Check sheet for the modelled part. Datum: model origin and axes. Units: mm. Face numbers are marked on the shaded views. A direction names the side the tool comes from. Round coordinates to 2 decimals unless told otherwise and drop trailing zeros. Write each loop counter-clockwise with the first axis right and the second up, starting at its lowest first coordinate (ties: lowest second). Pieces come first, ordered by that corner, then holes.
Item 1: Section check D-D, the plane y = 3.5. Record the cut outline in (x, z) (3 decimals), plus the area to 3 significant figures.
Item 2: Material ranges on line 1 along Z through (x, y) = (25.4, 4.25); line 2 along X through (y, z) = (4.25, -10); line 3 along Z through (x, y) = (12, 3.75), recorded low to high.
Item 3: Depth check by flat-ended pin: pin 1 (2 mm diameter, centred on x = 53.5, y = 5, fed in from -Z); pin 2 (3 mm diameter, centred on y = 2, z = -32.5, fed in from -X); pin 3 (1.9 mm diameter, centred on x = 13, y = 3, fed in from -Z). Enter the tip coordinate at first touch or a pass-through.
Item 4: Section check C-C, the plane x = 25.4. Record the cut outline in (y, z).
Item 5: Section check A-A, the plane x = 48.5. Record the cut outline in (y, z).
Item 6: Set-up check for the marked faces 1 and 2: record each of +Z, -Z, +X, -X, +Y, -Y from which the full face is reachable in a straight line by a thin tool's end or side.
Item 7: Section check B-B, the plane z = -19.05. Record the cut outline in (x, y), plus the area to 3 significant figures.
Item 8: Release check for a two-part mould opening along Z. For the marked faces 3, 4, 5 and 6 record: pulls with the +Z half, pulls with the -Z half, needs draft (parallel to the pull), parting line crosses it, or undercut.
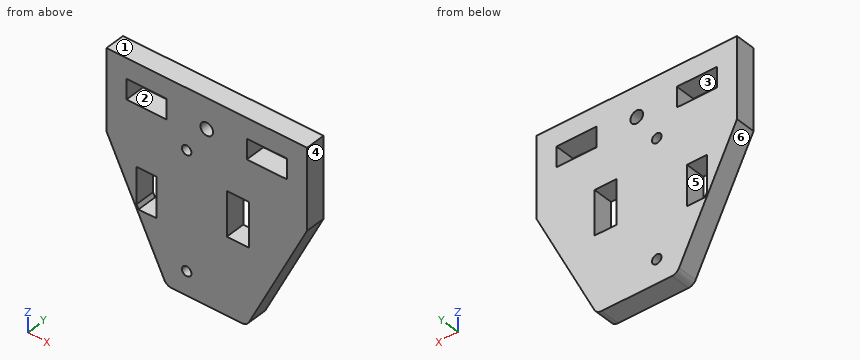
from build123d import *

# Parameters (mm, degrees)
SKETCH2_R               = 2
SKETCH2_R_2             = 1.5
SKETCH2_W               = 12.7
SKETCH2_H               = 6.35
SKETCH2_W_2             = 7
SKETCH2_H_2             = 13.97
BOSS_EXTRUDE1_DEPTH     = 6.35
CUT_EXTRUDE7_DEPTH      = 6.35
CUT_EXTRUDE8_DEPTH      = 1
CUT_EXTRUDE8_DEPTH_BACK = 6.35
CUT_EXTRUDE_THIN1_DEPTH = 6.35


with BuildPart() as part:
    # Sketch2 → Boss-Extrude1 (new body)
    with BuildSketch(Plane(origin=(0, 0, 0), x_dir=(1, 0, 0), z_dir=(0, 1, 0))):
        Polygon((0, 25.4), (25.4, 76.2), (38.1, 76.2), (63.5, 25.4), (63.5, 0), (0, 0), align=None)
        with Locations((31.75, 9.525)):
            Circle(SKETCH2_R, mode=Mode.SUBTRACT)
        with Locations((25.4, 19.05)):
            Circle(SKETCH2_R_2, mode=Mode.SUBTRACT)
        with Locations((25.4, 56.05)):
            Circle(SKETCH2_R_2, mode=Mode.SUBTRACT)
        with Locations((12.7, 9.525)):
            Rectangle(SKETCH2_W, SKETCH2_H, mode=Mode.SUBTRACT)
        with Locations((50.8, 9.525)):
            Rectangle(SKETCH2_W, SKETCH2_H, mode=Mode.SUBTRACT)
        with Locations((41.6, 32.385)):
            Rectangle(SKETCH2_W_2, SKETCH2_H_2, mode=Mode.SUBTRACT)
    extrude(amount=BOSS_EXTRUDE1_DEPTH)

    # Sketch3 → Cut-Extrude7 (cut)
    with BuildSketch(Plane(origin=(0, 6.35, 0), x_dir=(1, 0, 0), z_dir=(0, 1, 0))):
        Polygon((10.16, 44.45), (15.875, 44.45), (15.875, 31.75), (9.525, 31.75), (9.525, 43.18), align=None)
    extrude(amount=-CUT_EXTRUDE7_DEPTH, mode=Mode.SUBTRACT)

    # Sketch4 → Cut-Extrude8 (cut, two sides)
    with BuildSketch(Plane(origin=(0, 6.35, 0), x_dir=(1, 0, 0), z_dir=(0, 1, 0))) as cut_extrude8_sk:
        Polygon((-145.97325632, 63.5), (19.05, 63.5), (44.45, 63.5), (209.47325632, 63.5), (209.47325632, 393.54651264), (-145.97325632, 393.54651264), align=None)
    extrude(amount=CUT_EXTRUDE8_DEPTH, mode=Mode.SUBTRACT)
    extrude(cut_extrude8_sk.sketch, amount=-CUT_EXTRUDE8_DEPTH_BACK, mode=Mode.SUBTRACT)

    # Sketch5 → Cut-Extrude-Thin1 (cut)
    with BuildSketch(Plane(origin=(0, 6.35, 0), x_dir=(1, 0, 0), z_dir=(0, 1, 0))):
        with BuildLine():
            ThreePointArc((45.152038734, 62.095922533), (44.215550693, 63.120653053), (42.880193669, 63.5))
            Line((42.880193669, 63.5), (42.880193669, 66.04))
            ThreePointArc((42.880193669, 66.04), (45.550907718, 65.281306106), (47.423883799, 63.231845065))
            Line((47.423883799, 63.231845065), (45.152038734, 62.095922533))
        make_face()
        with BuildLine():
            ThreePointArc((20.619806331, 63.5), (19.284449307, 63.120653053), (18.347961266, 62.095922533))
            Line((18.347961266, 62.095922533), (16.076116201, 63.231845065))
            ThreePointArc((16.076116201, 63.231845065), (17.949092282, 65.281306106), (20.619806331, 66.04))
            Line((20.619806331, 66.04), (20.619806331, 63.5))
        make_face()
    extrude(amount=-CUT_EXTRUDE_THIN1_DEPTH, mode=Mode.SUBTRACT)


solid = part.part
Values found:
1. outline: (0, -25.4) - (18.348, -62.096) arc R2.54 ccw to (20.62, -63.5) - (42.88, -63.5) arc R2.54 ccw to (45.152, -62.096) - (63.5, -25.4) - (63.5, 0) - (0, 0) - close; hole (6.35, -12.7) - (19.05, -12.7) - (19.05, -6.35) - (6.35, -6.35) - close; hole (9.525, -43.18) - (10.16, -44.45) - (15.875, -44.45) - (15.875, -31.75) - (9.525, -31.75) - close; hole circle Ø3 at (25.4, -56.05); hole circle Ø3 at (25.4, -19.05); hole circle Ø4 at (31.75, -9.525); hole (38.1, -39.37) - (45.1, -39.37) - (45.1, -25.4) - (38.1, -25.4) - close; hole (44.45, -12.7) - (57.15, -12.7) - (57.15, -6.35) - (44.45, -6.35) - close
1. area: 2,940 mm2
2. line 1: z = -63.5 to -57.55, -54.55 to -20.55, -17.55 to 0
2. line 2: x = 0 to 6.35, 19.05 to 29.81, 33.69 to 44.45, 57.15 to 63.5
2. line 3: z = -49.4 to -44.45, -31.75 to -12.7, -6.35 to 0
3. pin 1: stops at z = -47.4
3. pin 2: stops at x = 2.8
3. pin 3: stops at z = -53.3
4. outline: (0, -63.5) - (6.35, -63.5) - (6.35, -57.55) - (0, -57.55) - close; (0, -54.55) - (6.35, -54.55) - (6.35, -20.55) - (0, -20.55) - close; (0, -17.55) - (6.35, -17.55) - (6.35, 0) - (0, 0) - close
5. outline: (0, -55.4) - (6.35, -55.4) - (6.35, -12.7) - (0, -12.7) - close; (0, -6.35) - (6.35, -6.35) - (6.35, 0) - (0, 0) - close
6. face 1: +Z, +X, -X, +Y, -Y
6. face 2: +Y, -Y
7. outline: (0, 0) - (23.9, 0) - (23.9, 6.35) - (0, 6.35) - close; (26.9, 0) - (63.5, 0) - (63.5, 6.35) - (26.9, 6.35) - close
7. area: 384 mm2
8. face 3: undercut
8. face 4: needs draft
8. face 5: undercut
8. face 6: pulls with the -Z half
